Read the model definition and answer for the solid it produces. Units are mm, in the model's axes. Face numbers are marked on the shaded views. A direction names the side the tool comes from. Give positions to 0.01 mm unless a question says otherwise; leave off trailing zeros. Write each loop counter-clockwise with the first axis right and the second up, starting at its lowest first coordinate (ties: lowest second). Pieces come first, ordered by that corner, then holes. Notation, with made-up numbers: (-2.5, 8) -> (24.5, 8) arc R21 cw to (24.5, 21) -> close; hole circle Ø4 at (-30.75, 8.5). An arc over 180 degrees is marked (long way). Answer as CSV lines item,"result". Start each with the question number.
1. The part is cut by section D-D, the plane z = 3.5. Determine the outline of the cut face in (x, y), and give its area (3 significant figures).
2. The part is cut by section C-C, the plane y = 5.5. Determine the outline of the cut face in (x, z).
3. The part is cut by section B-B, the plane y = -7.75. Determine the outline of the cut face in (x, z).
4. A tool of negligible diameter and unlimited length cuts with its end or side. For the marked faces 1, 2 and 3, from which of +Z, -Z, +X, -X, +Y, -Y can it reach the whole face along a straight path? Write none if from no direction.
5. Given pin 1 (3 mm diameter, centred on x = -45, z = 12, fed in from +Y); pin 2 (10 mm diameter, centred on y = 0.5, z = 4.5, fed in from -X); pin 3 (6 mm diameter, centred on y = 1.5, z = 10.5, fed in from +X); pin 4 (3.5 mm diameter, centred on x = -13.33, z = 10, fed in from -Y), each flat-ended and moving along its own axis, determine where each tip first touches the part or whether it passes through.
6. Find the intervals of material crossed by line 1 (X direction, y = 9, z = 8.5); line 2 (X direction, y = -7.5, z = 11.5); line 3 (X direction, y = -3.75, z = 1), in increasing order.
7. The part is cut by section A-A, the plane x = -25.5. Determine the outline of the cut face in (y, z).
from build123d import *

# Parameters (mm, degrees)
F1_DEPTH = 20
F2_R     = 1.5
F3_DEPTH = 20
F4_W     = 2.8
F4_H     = 6
F5_DEPTH = 7.5
F6_R     = 2.25
F7_DEPTH = 6


with BuildPart() as f1:
    # F0 (on Top) → F1 (new body)
    with BuildSketch(Plane.XY):
        with BuildLine():
            Line((-38.333333, 14.652778), (-38.333333, -5.347222))
            Line((-38.333333, -5.347222), (-18.333333, -5.347222))
            Line((-18.333333, -5.347222), (-18.333333, 14.652778))
            Line((-18.333333, 14.652778), (-27.583333, 14.652778))
            Line((-27.583333, 14.652778), (-27.583333, 8.683597))
            ThreePointArc((-27.583333, 8.683597), (-25.18016, 7.273369), (-24.233333, 4.652778))
            ThreePointArc((-24.233333, 4.652778), (-30.953925, 1.499605), (-29.083333, 8.683597))
            Line((-29.083333, 8.683597), (-29.083333, 14.652778))
            Line((-29.083333, 14.652778), (-38.333333, 14.652778))
        make_face()
        Polygon((-48.333333, -5.347222), (-48.333333, -11.347222), (-8.333333, -11.347222), (-8.333333, -5.347222), (-18.333333, -5.347222), (-38.333333, -5.347222), align=None)
    extrude(amount=F1_DEPTH)

    # F2 (on face) → F3 (cut)
    with BuildSketch(Plane(origin=(-38.333333, 0, 0), x_dir=(0, -1, 0), z_dir=(-1, 0, 0))):
        with Locations((-11.152778, 10)):
            Circle(F2_R)
    extrude(amount=-F3_DEPTH, mode=Mode.SUBTRACT)

    # F4 (on face) → F5 (cut)
    with BuildSketch(Plane(origin=(0, 14.652778, 0), x_dir=(-1, 0, 0), z_dir=(0, 1, 0))):
        with Locations((20.733333, 10)):
            Rectangle(F4_W, F4_H)
    extrude(amount=-F5_DEPTH, mode=Mode.SUBTRACT)

    # F6 (on face) → F7 (cut)
    with BuildSketch(Plane(origin=(0, -5.347222, 0), x_dir=(-1, 0, 0), z_dir=(0, 1, 0))):
        with Locations((43.333333, 10)):
            Circle(F6_R)
        with Locations((13.333333, 10)):
            Circle(F6_R)
    extrude(amount=-F7_DEPTH, mode=Mode.SUBTRACT)


solid = f1.part
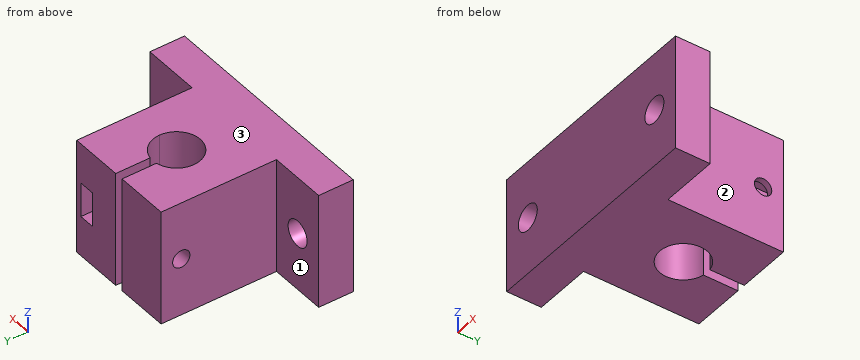
Results found:
1,outline,"(-48.33, -11.35) -> (-8.33, -11.35) -> (-8.33, -5.35) -> (-18.33, -5.35) -> (-18.33, 14.65) -> (-27.58, 14.65) -> (-27.58, 8.68) arc R4.1 cw to (-24.23, 4.65) arc R4.1 cw (long way) to (-29.08, 8.68) -> (-29.08, 14.65) -> (-38.33, 14.65) -> (-38.33, -5.35) -> (-48.33, -5.35) -> close"
1,area,"578 mm²"
2,outline,"(-38.33, 0) -> (-32.34, 0) -> (-32.34, 20) -> (-38.33, 20) -> close; (-24.32, 0) -> (-18.33, 0) -> (-18.33, 20) -> (-24.32, 20) -> close"
3,outline,"(-48.33, 0) -> (-8.33, 0) -> (-8.33, 20) -> (-48.33, 20) -> close; hole circle Ø4.5 at (-43.33, 10); hole circle Ø4.5 at (-13.33, 10)"
4,face 1,"+Z, -Z, -X, +Y"
4,face 2,"+Z, -Z, +X, +Y"
4,face 3,"+Z, +X, -X, +Y, -Y"
5,pin 1,"stops at y = -5.35"
5,pin 2,"stops at x = -38.33"
5,pin 3,"stops at x = -18.33"
5,pin 4,"passes through"
6,line 1,"x = -38.33 to -29.08, -27.58 to -22.13, -19.33 to -18.33"
6,line 2,"x = -48.33 to -45.01, -41.66 to -15.01, -11.66 to -8.33"
6,line 3,"x = -38.33 to -18.33"
7,outline,"(-11.35, 0) -> (1.69, 0) -> (1.69, 20) -> (-11.35, 20) -> close; (7.62, 0) -> (14.65, 0) -> (14.65, 20) -> (7.62, 20) -> close; hole circle Ø3 at (11.15, 10)"
